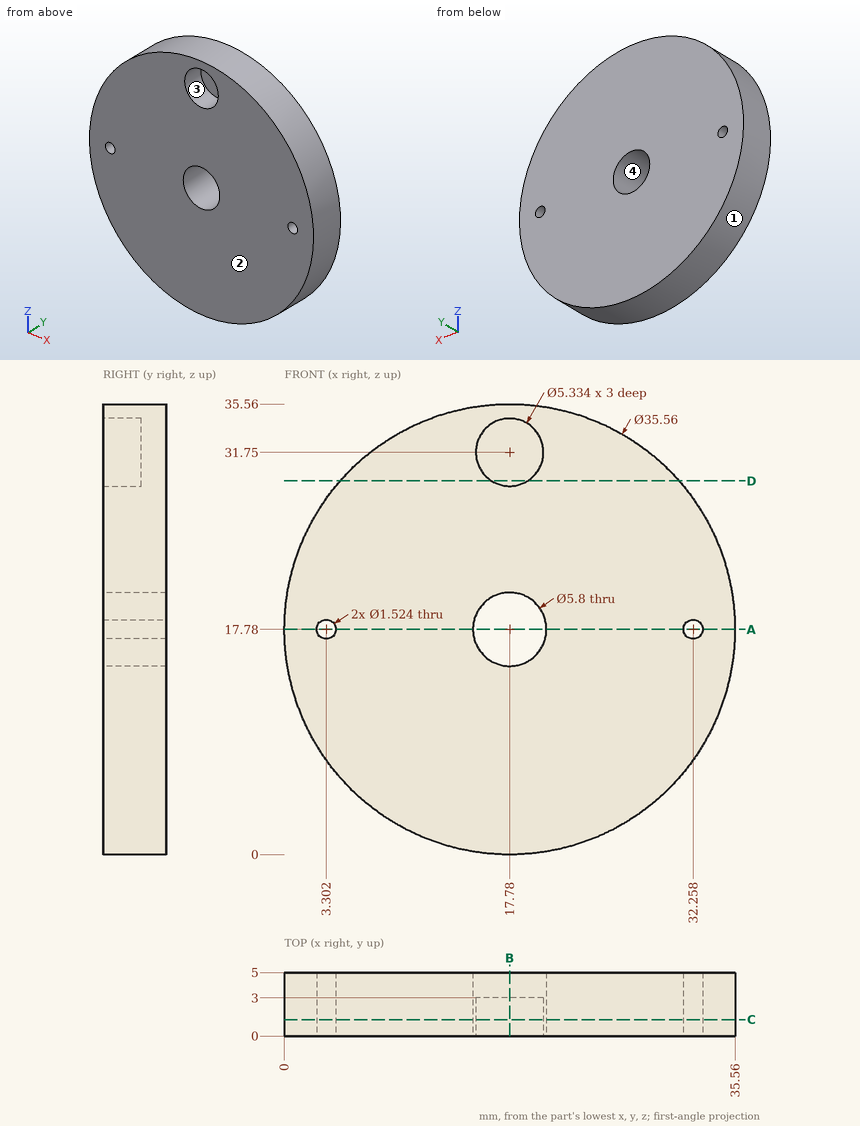
Answer from the drawing. Dimensions are ordinates in mm from the lowest x, y and z of the part. Give positions to 0.01 mm unless a question says otherwise; leave off trailing zeros. Order: outer loops, then holes, each group sorted by start corner. A loop starts at its lowest first (then second) coordinate and runs counter-clockwise, first axis right, second up. Notation, with made-up numbers: (-34, 43.25) -> (13, 43.25) arc R22 cw to (13, 71.25) -> close; hole circle Ø11 at (24.25, -4.75). An arc over 180 degrees is marked (long way). Answer as a JSON object with one key per item and string values. Group by question number.
1. The mould has two halves that part along X. Classify the marked faces 1, 2, 3 and 4: released by +X, released by -X, zero draft, split by the parting line, or undercut.
2. Section C-C on y = 1.3 is taken. Determine the outline of the cut face in (x, z), plus the area to 3 significant figures.
3. Flat-ended cylindrical pins translate along their axes: pin 1 Ø3 at (x, y) = (23, 1.5) entering from -Z; pin 2 Ø1.5 at (y, z) = (2.5, 28.5) entering from +X; pin 3 Ø3 at (x, y) = (29, 4) entering from +Z. Find the tip coordinate at first contact, or state that the pin passes through.
4. Section A-A on z = 17.78 is taken. Determine the outline of the cut face in (x, y), plus the area to 3 significant figures.
5. Section B-B on x = 17.78 is taken. Determine the outline of the cut face in (y, z).
6. Section D-D on z = 29.5 is taken. Determine the outline of the cut face in (x, y), plus the area to 3 significant figures.
7. Consider line 1 along X through (y, z) = (1.8, 17.78); line 2 along Y through (x, z) = (17, 30); line 3 along X through (y, z) = (3.65, 19). Determine where each line is inside the solid, lowest interval first. Write a range as [from, to].
Result sheet:
{
 "1": {"face 1": "split by the parting line", "face 2": "zero draft", "face 3": "undercut", "face 4": "undercut"},
 "2": {"outline": "circle Ø35.56 at (17.78, 17.78); hole circle Ø1.52 at (3.3, 17.78); hole circle Ø5.8 at (17.78, 17.78); hole circle Ø5.33 at (17.78, 31.75); hole circle Ø1.52 at (32.26, 17.78)", "area": "941 mm^2"},
 "3": {"pin 1": "stops at z = 0.39", "pin 2": "stops at x = 32.5", "pin 3": "stops at z = 32.67"},
 "4": {"outline": "(0, 0) -> (2.54, 0) -> (2.54, 5) -> (0, 5) -> close; (4.06, 0) -> (14.88, 0) -> (14.88, 5) -> (4.06, 5) -> close; (20.68, 0) -> (31.5, 0) -> (31.5, 5) -> (20.68, 5) -> close; (33.02, 0) -> (35.56, 0) -> (35.56, 5) -> (33.02, 5) -> close", "area": "134 mm^2"},
 "5": {"outline": "(0, 0) -> (5, 0) -> (5, 14.88) -> (0, 14.88) -> close; (0, 20.68) -> (5, 20.68) -> (5, 35.56) -> (0, 35.56) -> (0, 34.42) -> (3, 34.42) -> (3, 29.08) -> (0, 29.08) -> close"},
 "6": {"outline": "(4.41, 0) -> (16.35, 0) -> (16.35, 3) -> (19.21, 3) -> (19.21, 0) -> (31.15, 0) -> (31.15, 5) -> (4.41, 5) -> close", "area": "125 mm^2"},
 "7": {"line 1": "x = [0, 2.54], [4.06, 14.88], [20.68, 31.5], [33.02, 35.56]", "line 2": "y = [3, 5]", "line 3": "x = [0.04, 15.15], [20.41, 35.52]"}
}
